Autodesk Inventor part; units mm, degrees
ref_plane "YZ Plane" through (0, 0, 0) normal (1, 0, 0) x (0, 1, 0)
ref_plane "XZ Plane" through (0, 0, 0) normal (0, 1, 0) x (-1, 0, 0)
ref_plane "XY Plane" through (0, 0, 0) normal (0, 0, 1) x (1, 0, 0)
sketch "Sketch1" plane through (0, 0, 0) normal (0, 0, 1) x (1, 0, 0)
  line L0 (-13, 12) -> (13, 12)
  line L1 (13, 12) -> (13, -12)
  line L2 (13, -12) -> (-13, -12)
  line L3 (-13, -12) -> (-13, 12)
  line L4 (-13, 3.25) -> (-15, 3.25)
  line L5 (-15, 3.25) -> (-15, -3.25)
  line L6 (-15, -3.25) -> (-13, -3.25)
  line L7 (-13, -3.25) -> (-13, 3.25)
  line L8 (13, 3.25) -> (15, 3.25)
  line L9 (15, 3.25) -> (15, -3.25)
  line L10 (15, -3.25) -> (13, -3.25)
  line L11 (13, -3.25) -> (13, 3.25)
  line L12 (-25.4, 25.4) -> (25.4, 25.4)
  line L13 (25.4, 25.4) -> (25.4, -25.4)
  line L14 (25.4, -25.4) -> (-25.4, -25.4)
  line L15 (-25.4, -25.4) -> (-25.4, 25.4)
  circle A0 centre (0, 0) radius 7.1437
  circle A1 centre (-3, 12) radius 1.5
  line L16 (-13, 8) -> (-9, 12)
  line L17 (9, 12) -> (13, 8)
  line L18 (13, -8) -> (9, -12)
  line L19 (-13, -8) -> (-9, -12)
  line L20 (-13, 3.25) -> (13, 3.25)
  line L21 (13, -3.25) -> (-13, -3.25)
  point P0 (-14, 3.25)
  point P1 (14, 3.25)
  point P2 (-14, -3.25)
  point P3 (14, -3.25)
  point P4 (-20.32, 20.32)
  point P5 (20.32, 20.32)
  point P6 (20.32, -20.32)
  point P7 (-20.32, -20.32)
  dimension "d0" = 24
  dimension "d1" = 12
  dimension "d2" = 26
  dimension "d3" = 13
  dimension "d4" = 2
  dimension "d5" = 6.5
  dimension "d6" = 3.25
  dimension "d7" = 2
  dimension "d8" = 14.2875
  dimension "d9" = 50.8
  dimension "d10" = 25.4
  dimension "d11" = 50.8
  dimension "d12" = 25.4
  dimension "d13" = 3
  dimension "d14" = 10
  dimension "d15" = 4
  dimension "d16" = 4
  dimension "d17" = 4
  dimension "d18" = 4
  dimension "d19" = 4
  dimension "d20" = 5.08
  dimension "d21" = 5.08
  dimension "d22" = 5.08
  dimension "d23" = 5.08
  dimension "d34" = 40.64
  dimension "d35" = 40.64
extrude "Extrusion1" add sketch "Sketch1" against normal blind 12.7 contours L0 L16 L3 | L0 L1 L17 | L19 L2 L3 | L18 L1 L2 | L12 L13 L14 L15
fillet "Fillet1" radius 3.175 4 edges at (-13, -3.25, -6.35) (-13, 3.25, -6.35) (13, 3.25, -6.35) (13, -3.25, -6.35)
extrude "Extrusion2" add sketch "Sketch1" along normal blind 1.5875 contours L0 L16 L3 | L0 A1 L17 L1 L20 A0 L3 L16 | A1 L0 | L0 A1 | L21 A0 L1 L18 L2 L19 L3 | L0 L1 L17 | L19 L2 L3 | L18 L1 L2 | L12 L13 L14 L15
hole "Hole1" at (-20.32, 20.32, 0) at (20.32, 20.32, 0) at (20.32, -20.32, 0) at (-20.32, -20.32, 0) direction (0, 0, -1) diameter 4.1656 end through all
thread "Thread1"
thread "Thread2"
thread "Thread3"
thread "Thread4"
hole "Hole2" at (20.32, 20.32, 0) at (-20.32, 20.32, 0) at (-20.32, -20.32, 0) at (20.32, -20.32, 0) direction (0, 0, 1) diameter 4.1656 end through all
fillet "Fillet2" radius 6.35 4 edges at (25.4, 25.4, -5.5563) (-25.4, 25.4, -5.5562) (-25.4, -25.4, -5.5562) (25.4, -25.4, -5.5563)
equation "\"d7\" = d4"
equation "\"d16\" = d15"
equation "\"d17\" = d15"
equation "\"d18\" = d15"
equation "\"d19\" = d15"
properties part number "BD gearbox mount block 2"
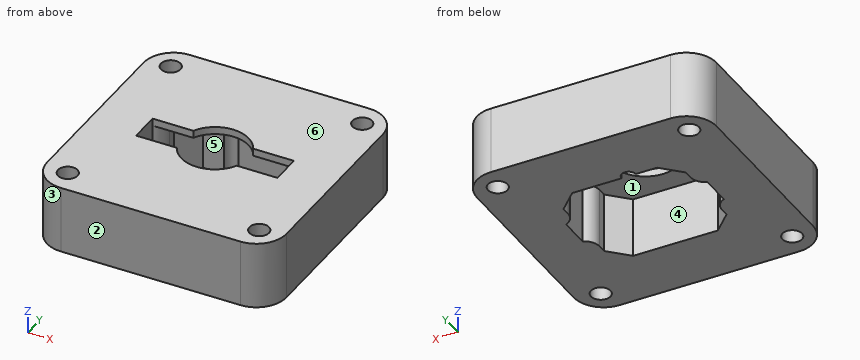
Verification items for the finished model (mm, model axes). Face numbers are marked on the shaded views. A direction names the side the tool comes from. Coordinates: 2 decimals unless noted, no trailing zeros. Loops run counter-clockwise (first coordinate to the right, second up) from the corner with the lowest first, then second, coordinate; pieces in that order, holes last. Notation, with made-up numbers: (17.5, 32.5) -> (76.5, 32.5) arc R17 cw to (76.5, 64.5) -> close; hole circle Ø5 at (23.5, 44). An arc over 180 degrees is marked (long way). Answer as CSV lines item,"result".
1) Cross-section at C-C, the plane x = -21. Record the cut outline in (y, z), then the cut area to 3 significant figures.
Found:
outline,"(-25.09, -12.7) -> (-22.29, -12.7) -> (-22.29, 1.59) -> (-25.09, 1.59) -> close; (-18.35, -12.7) -> (18.35, -12.7) -> (18.35, 1.59) -> (-18.35, 1.59) -> close; (22.29, -12.7) -> (25.09, -12.7) -> (25.09, 1.59) -> (22.29, 1.59) -> close"
area,"605 mm2"
2) Cross-section at B-B, the plane z = -6. Count the separate pieces of the cut face and the enclosed holes in it, then the cut area to 3 significant figures.
Found:
separate pieces,"1"
enclosed holes,"5"
area,"1,860 mm2"
3) Depth check by flat-ended pin: pin 1 (8 mm diameter, centred on x = -3, y = -11.5, fed in from -Z); pin 2 (2.5 mm diameter, centred on x = -20.32, y = -20.32, fed in from +Z); pin 3 (5 mm diameter, centred on x = -5, y = 7.5, fed in from -Z). Enter the tip coordinate at first touch or a pass-through.
Found:
pin 1,"stops at z = -12.7"
pin 2,"passes through"
pin 3,"stops at z = 0"
4) Cross-section at A-A, the plane x = 10.5. Record the cut outline in (y, z), then the cut area to 3 significant figures.
Found:
outline,"(-25.4, -12.7) -> (-10.5, -12.7) -> (-10.5, 0) -> (-3.25, 0) -> (-3.25, 1.59) -> (-25.4, 1.59) -> close; (3.25, 0) -> (10.5, 0) -> (10.5, -12.7) -> (25.4, -12.7) -> (25.4, 1.59) -> (3.25, 1.59) -> close"
area,"449 mm2"
5) Cross-section at D-D, the plane y = -20.32. Record the cut outline in (x, z), then the cut area to 3 significant figures.
Found:
outline,"(-25.27, -12.7) -> (-22.4, -12.7) -> (-22.4, 1.59) -> (-25.27, 1.59) -> close; (-18.24, -12.7) -> (18.24, -12.7) -> (18.24, 1.59) -> (-18.24, 1.59) -> close; (22.4, -12.7) -> (25.27, -12.7) -> (25.27, 1.59) -> (22.4, 1.59) -> close"
area,"603 mm2"
6) Tool access check on the marked faces 5 and 6. Record the directions out of +Z, -Z, +X, -X, +Y, -Y that give a thin tool (end or side, any length) a straight path to the whole face; none if there is none.
Found:
face 5,"-Z"
face 6,"+Z, +X, -X, +Y, -Y"
7) Release check for a two-part mould opening along X. For the marked faces 1, 2, 3 and 4 record: +X half, -X half, draft (parallel to the pull), parting line (faces both ways), or undercut.
Found:
face 1,"undercut"
face 2,"draft"
face 3,"-X half"
face 4,"undercut"
8) Thickness scan on L1, parallel to Y at x = -8, z = -3.75; L2, parallel to X at y = 21, z = -3.5; L3, parallel to Y at x = 20.32, z = -6.5. Record the ranges inside material, lowest first. Write a range as from..to.
Found:
L1,"y = -25.4..-12, 12..25.4"
L2,"x = -25.09..-22.29, -18.35..18.35, 22.29..25.09"
L3,"y = -25.27..-22.4, -18.24..18.24, 22.4..25.27"
